Geometry check sheet. Reference: the model listing, model coordinates, mm. A direction names the side the tool comes from. Round coordinates to 2 decimals unless told otherwise and drop trailing zeros. Loops run counter-clockwise (first coordinate to the right, second up) from the corner with the lowest first, then second, coordinate; pieces in that order, holes last. Notation, with made-up numbers: (-18, -4) - (38, -4) arc R21 ccw to (38, 16) - close; hole circle Ø1 at (17.25, -7.5). An arc over 180 degrees is marked (long way). Answer as CSV lines item,"result". Start each with the question number.
1) Depth check by flat-ended pin: P1, Ø12.5, axis at x = -4.5, y = 0, coming from the +Z side; P2, Ø5, axis at y = 35, z = 9, coming from the -X side; P3, Ø12, axis at y = 21.5, z = 22.5, coming from the +X side; P4, Ø7.5, axis at x = 0, y = 38.1, coming from the +Z side. Enter the tip coordinate at first touch or a pass-through.
2) Access from +Z, -Z, +X, -X, +Y, -Y to the whole of each face (thin tool, end or side, straight path). Record for faces 5 (the cylindrical face through (6.057, -36.193, 12.878)), 6 (the cylindrical face through (-2.75, 12.4, 37.92)).
3) Thickness scan on line 1 along Y through (x, z) = (0, 20); line 2 along Y through (x, z) = (0, 30); line 3 along Z through (x, y) = (-42, -9). Record the ranges inside material, lowest first.
4) Draft check along Y on faces 1 (the cylindrical face through (31.756, 0.279, 12.878)), 2 (the flat face through (5, 12, 50.8)), 3 (the cylindrical face through (-13.77, 61.99, 12.52)), 4 (the cylindrical face through (-1.38, 31.9, 12.88)). Enter one of: released by +Y, released by -Y, zero draft, split by the parting line, or undercut.
5) Cross-section at A-A on y = 0. Record the boundary of the cut face in (x, z), and give its area (3 significant figures).
6) Cross-section at B-B on y = 38.1. Record the boundary of the cut face in (x, z), and give its area (3 significant figures).
7) Cross-section at D-D on z = 13. Record the boundary of the cut face in (x, y), and give its area (3 significant figures).
Autodesk Inventor part; units mm, degrees
ref_plane "YZ Plane" through (0, 0, 0) normal (1, 0, 0) x (0, 1, 0)
ref_plane "XZ Plane" through (0, 0, 0) normal (0, 1, 0) x (-1, 0, 0)
ref_plane "XY Plane" through (0, 0, 0) normal (0, 0, 1) x (1, 0, 0)
sketch "Sketch1" plane through (0, 0, 0) normal (0, 0, 1) x (1, 0, 0)
  circle A0 centre (0, 0) radius 63.5
  dimension "d0" = 127
extrude "Extrusion1" add sketch "Sketch1" along normal blind 25.4
sketch "Sketch2" plane through (0, 0, 25.4) normal (0, 0, 1) x (1, 0, 0)
  circle A0 centre (0, 0) radius 25.4
  circle A1 centre (0, 0) radius 12.7
  circle A2 centre (0, -38.1) radius 6.35
  circle A3 centre (-38.1, 0) radius 6.35
  dimension "d3" = 50.8
  dimension "d4" = 25.4
  dimension "d5" = 12.7
  dimension "d6" = 38.1
  dimension "d7" = 12.7
  dimension "d8" = 38.1
sketch "Sketch3" plane through (0, 0, 25.4) normal (0, 0, 1) x (1, 0, 0)
  circle A0 centre (38.1, 0) radius 6.35
  circle A1 centre (0, 38.1) radius 6.35
  point P0 (0, 0)
  dimension "d9" = 12.7
  dimension "d10" = 38.1
  dimension "d11" = 12.7
  dimension "d12" = 38.1
extrude "Extrusion2" add sketch "Sketch2" along normal blind 25.4 contours A0
sketch "Sketch4" plane through (0, 0, 25.4) normal (0, 0, 1) x (1, 0, 0)
  circle A0 centre (-38.1, 0) radius 6.35
  circle A1 centre (0, -38.1) radius 6.35
  point P0 (0, 0)
  dimension "d15" = 12.7
  dimension "d16" = 38.1
  dimension "d17" = 12.7
  dimension "d18" = 38.1
extrude "Extrusion3" cut sketch "Sketch3" against normal blind 381 contours A1
extrude "Extrusion4" cut sketch "Sketch4" against normal blind 381
sketch "Sketch5" plane through (0, 0, 25.4) normal (0, 0, 1) x (1, 0, 0)
  circle A0 centre (38.1, 0) radius 6.35
  point P0 (0, 0)
  dimension "d23" = 12.7
  dimension "d24" = 38.1
extrude "Extrusion5" cut sketch "Sketch5" against normal blind 381
properties part number "test 2018 1"
Answer block:
1,P1,"stops at z = 25.4"
1,P2,"stops at x = -54.55"
1,P3,"stops at x = 61.58"
1,P4,"passes through"
2,face 5,"+Z, -Z"
2,face 6,"+Z"
3,line 1,"y = -63.5 to -44.45, -31.75 to 31.75, 44.45 to 63.5"
3,line 2,"y = -25.4 to -12.7, 12.7 to 25.4"
3,line 3,"z = 0 to 25.4"
4,face 1,"undercut"
4,face 2,"zero draft"
4,face 3,"split by the parting line"
4,face 4,"undercut"
5,outline,"(-63.5, 0) - (-44.45, 0) - (-44.45, 25.4) - (-63.5, 25.4) - close; (-31.75, 0) - (31.75, 0) - (31.75, 25.4) - (25.4, 25.4) - (25.4, 50.8) - (12.7, 50.8) - (12.7, 25.4) - (-12.7, 25.4) - (-12.7, 50.8) - (-25.4, 50.8) - (-25.4, 25.4) - (-31.75, 25.4) - close; (44.45, 0) - (63.5, 0) - (63.5, 25.4) - (44.45, 25.4) - close"
5,area,"3,230 mm^2"
6,outline,"(-50.8, 0) - (-6.35, 0) - (-6.35, 25.4) - (-50.8, 25.4) - close; (6.35, 0) - (50.8, 0) - (50.8, 25.4) - (6.35, 25.4) - close"
6,area,"2,260 mm^2"
7,outline,"circle Ø127 at (0, 0); hole circle Ø12.7 at (-38.1, 0); hole circle Ø12.7 at (0, -38.1); hole circle Ø12.7 at (0, 38.1); hole circle Ø12.7 at (38.1, 0)"
7,area,"12,200 mm^2"
